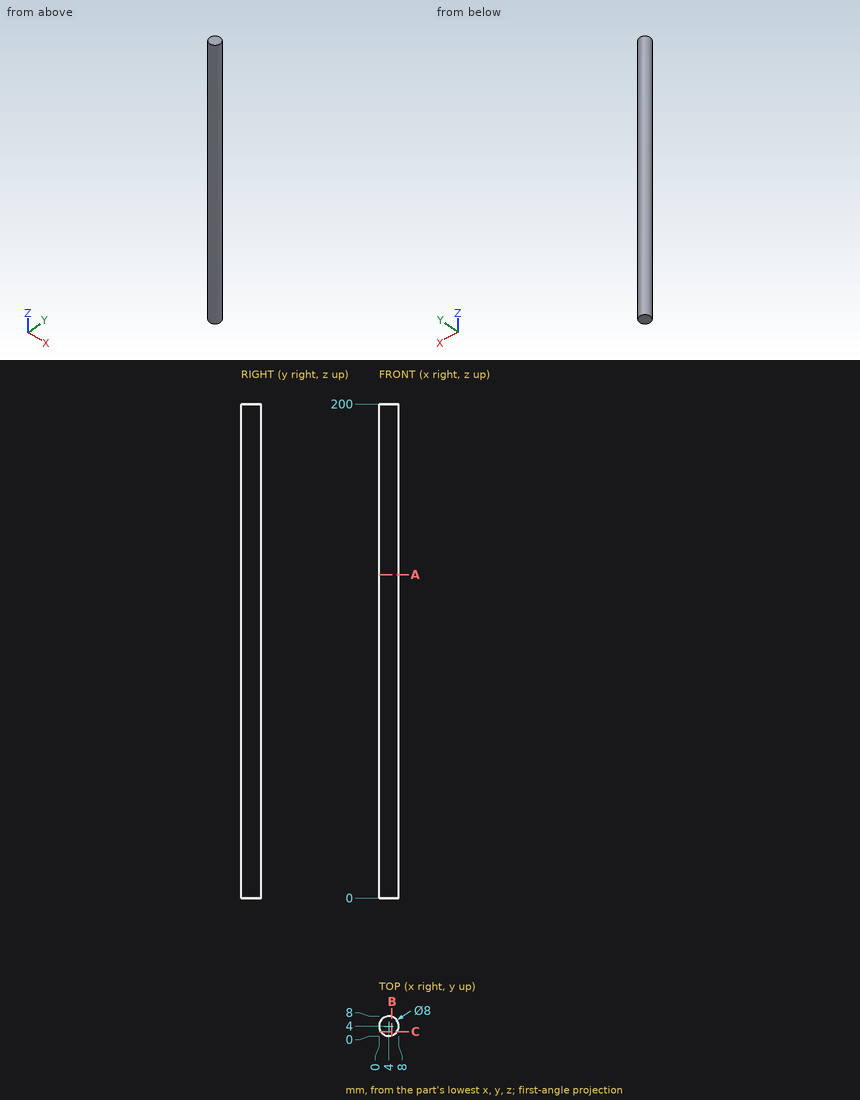
Input: dimensioned drawing with shaded views. Units: mm. Origin: part minimum x, y, z. Give positions to 0.01 mm unless a question says otherwise; leave off trailing zeros. Write each loop counter-clockwise with the first axis right and the second up, starting at its lowest first coordinate (ties: lowest second). Pieces come first, ordered by that corner, then holes.
Q1. First-contact query: P1, Ø4, axis at x = 6, z = 137.5, coming from the -Y side; P2, Ø2, axis at x = 6.5, z = 95.5, coming from the +Y side. Flat tips, straight axial feed; report the tip coordinate or a pass-through.
Q2. Section A-A, the plane z = 131. Output: boundary loops of the cut face in (x, y).
Q3. Section C-C, the plane y = 1.75. Output: boundary loops of the cut face in (x, z).
Q4. Section B-B, the plane x = 5.25. Output: boundary loops of the cut face in (y, z), plus the area to 3 significant figures.
Q5. Material intervals for probe 1 along Y at (x, z) = (4.5, 139.5); probe 2 along Y at (x, z) = (2.25, 82), sorted ascending.
Filled in:
1. P1: stops at y = 0
1. P2: stops at y = 7.71
2. outline: circle Ø8 at (4, 4)
3. outline: (0.69, 0) - (7.31, 0) - (7.31, 200) - (0.69, 200) - close
4. outline: (0.2, 0) - (7.8, 0) - (7.8, 200) - (0.2, 200) - close
4. area: 1,520 mm2
5. probe 1: y = 0.03 to 7.97
5. probe 2: y = 0.4 to 7.6
